from build123d import *


with BuildPart() as part:
    # 草图1 → 旋转1 (revolve)
    with BuildSketch(Plane.XY):
        with BuildLine():
            Line((2, 17), (3, 17))
            Line((3, 17), (3, 11.587964483))
            ThreePointArc((3, 11.587964483), (3.757997248, 9.757997248), (5.587964483, 9))
            Line((5.587964483, 9), (8.5, 9))
            Line((8.5, 9), (8.5, 5.1))
            Line((8.5, 5.1), (4.4, 5.1))
            Line((4.4, 5.1), (4.4, 4.5))
            Line((4.4, 4.5), (1.1, 4.5))
            Line((1.1, 4.5), (1.1, 5.1))
            Line((1.1, 5.1), (-3, 5.1))
            Line((-3, 5.1), (-3, 17))
            Line((-3, 17), (-2, 17))
            ThreePointArc((-2, 17), (0, 15), (2, 17))
        make_face()
    revolve(axis=Axis((0, 0, 0), (1, 0, 0)))


solid = part.part
Could you check a few things on this model? Use its own coordinates, in mm. A direction names the side the tool comes from. Coordinates: 2 decimals unless noted, no trailing zeros. Order: outer loops, then holes, each group sorted by start corner. A loop starts at its lowest first (then second) coordinate and runs counter-clockwise, first axis right, second up.
Q1. Will these pins go through, and if not, where does the flat tip stop? pin 1 (5 mm diameter, centred on x = 7.5, z = -3, fed in from -Y); pin 2 (5 mm diameter, centred on x = -1, y = -13, fed in from -Z); pin 3 (6 mm diameter, centred on x = 3, y = 5, fed in from +Z).
Q2. Please list where these lines run through material, in increasing order: L1, parallel to Z at x = 6.25, y = 0; L2, parallel to Z at x = 2.6, y = 0; L3, parallel to X at y = 4, z = -15.5.
Q3. Which directions (+Z, -Z, +X, -X, +Y, -Y) give clear straight access to the entire face, cutting with the end or side of a thin tool? Please do faces 4 (the cylindrical face through (-1, 2.4, -4.5)), 5 (the flat face through (-3, -4, 4)).
Q4. Thinking about a two-plate mould opening in Y: for faces 1 (the flat face through (3, -4, -11.1)), 2 (the cylindrical face through (6.4, 2.4, -4.5)), 3 (the cylindrical face through (7.064, -1.172, 8.923)), which applies, released by +Y, released by -Y, zero draft, split by the parting line, or undercut?
Q5. Suppose I cut it at A-A on z = 0. Please give me the cut outline in (x, y), and give its area (3 significant figures).
Q6. Suppose I cut it at C-C on x = -1.25. Please give me the cut outline in (y, z).
Answer:
1. pin 1: stops at y = -8.99
1. pin 2: stops at z = -13.2
1. pin 3: stops at z = 16.88
2. L1: z = -9 to -5.1, 5.1 to 9
2. L2: z = -17 to -4.5, 4.5 to 17
2. L3: x = -3 to -1.74, 1.74 to 3
3. face 4: -X
3. face 5: +Z, -Z, -X, +Y, -Y
4. face 1: zero draft
4. face 2: undercut
4. face 3: split by the parting line
5. outline: (-3, -17) - (-2, -17) arc R2 cw to (2, -17) - (3, -17) - (3, -11.59) arc R2.59 cw to (5.59, -9) - (8.5, -9) - (8.5, -5.1) - (4.4, -5.1) - (4.4, -4.5) - (1.1, -4.5) - (1.1, -5.1) - (-3, -5.1) - close; (-3, 5.1) - (1.1, 5.1) - (1.1, 4.5) - (4.4, 4.5) - (4.4, 5.1) - (8.5, 5.1) - (8.5, 9) - (5.59, 9) arc R2.59 cw to (3, 11.59) - (3, 17) - (2, 17) arc R2 cw to (-2, 17) - (-3, 17) - close
5. area: 180 mm2
6. outline: circle Ø30.88 at (0, 0); hole circle Ø10.2 at (0, 0)
